from build123d import *

# Parameters (mm, degrees)
F0_R     = 12.5
F0_W     = 5
F0_H     = 20
F1_DEPTH = 25
F2_R     = 15
F3_R     = 5
F4_R     = 2.5
F5_DEPTH = 5
F6_SIZE  = 0.5


with BuildPart() as f1:
    # F0 (on Top) → F1 (new body)
    with BuildSketch(Plane.XY):
        with BuildLine():
            ThreePointArc((-15, 0), (0, -15), (15, 0))
            ThreePointArc((15, 0), (5.352331, 14.012585), (-11.18034, 10))
            ThreePointArc((-11.18034, 10), (-14.012585, 5.352331), (-15, 0))
        make_face()
        Circle(F0_R, mode=Mode.SUBTRACT)
        with BuildLine():
            ThreePointArc((-15, 0), (-14.012585, 5.352331), (-11.18034, 10))
            Line((-11.18034, 10), (-20, 10))
            Line((-20, 10), (-20, 0))
            Line((-20, 0), (-15, 0))
        make_face()
        with Locations((-17.5, -10)):
            Rectangle(F0_W, F0_H)
    extrude(amount=F1_DEPTH)

    # F2
    f2_edges = [f1.edges().sort_by_distance(p)[0] for p in [
        (-11.18034, 10, 12.5),
    ]]
    fillet(f2_edges, radius=F2_R)

    # F3
    f3_edges = [f1.edges().sort_by_distance(p)[0] for p in [
        (-20, 10, 12.5),
    ]]
    fillet(f3_edges, radius=F3_R)

    # F4 (on face) → F5 (cut)
    with BuildSketch(Plane(origin=(-20, 0, 0), x_dir=(0, -1, 0), z_dir=(-1, 0, 0))):
        with Locations((15, 12.5)):
            Circle(F4_R)
    extrude(amount=-F5_DEPTH, mode=Mode.SUBTRACT)

    # F6
    f6_edges = [f1.edges().sort_by_distance(p)[0] for p in [
        (-12.5, 0, 0),
        (-12.5, 0, 25),
    ]]
    chamfer(f6_edges, length=F6_SIZE)


solid = f1.part
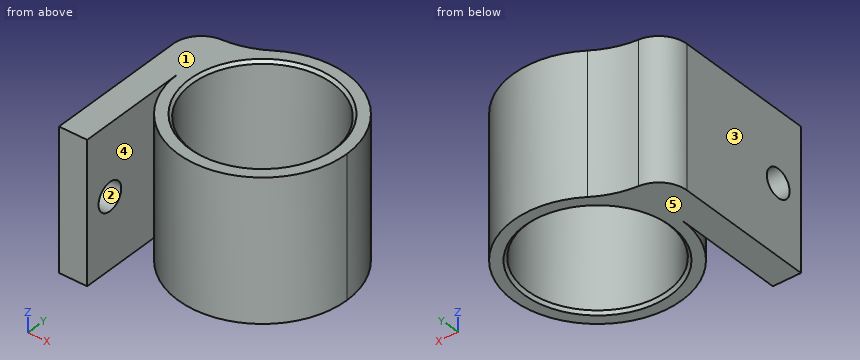
Design review of the part built by this model. Coordinates are the model's own, in mm. Face numbers are marked on the shaded views. A direction names the side the tool comes from. Give positions to 0.01 mm unless a question says otherwise; leave off trailing zeros. Loops run counter-clockwise (first coordinate to the right, second up) from the corner with the lowest first, then second, coordinate; pieces in that order, holes last. Notation, with made-up numbers: (19, -38.75) -> (67, -38.75) arc R6 ccw to (67, -33.75) -> close; hole circle Ø5 at (86.25, 28.5). An arc over 180 degrees is marked (long way). One line per question, with ' | ' between items. Start each with the question number.
(1) Insertion check: P1, Ø4, axis at x = -6, z = 5, coming from the -Y side; P2, Ø1.5, axis at x = -0.5, y = -12, coming from the -Z side; P3, Ø4, axis at y = -15, z = 12.5, coming from the +X side. Each pin has a flat end and moves straight along its axis. Give the tip position at first contact, or say it passes through.
(2) For the marked faces 1 and 2, list the 3-axis set-ups (+Z, -Z, +X, -X, +Y, -Y) from which the entire face can be reached by the end or side of a thin tool; tool diameter is ignored.
(3) For line 1 (Z direction, x = -18.45, y = -15); line 2 (Y direction, x = 0, z = 9); line 3 (X direction, y = 5.5, z = 18.5), list the stretches that pass through material, from the lowest coordinate up.
(4) Draft analysis for pull direction X (two halves, no side actions). For the marked faces 3, 4 and 5, state which applies: +X half, -X half, draft (parallel to the pull), parting line (faces both ways), or undercut.
(5) We need section A-A (x = 0). State the section outline as (y, z) points, and give its area (4 significant figures).
(6) We need section B-B (z = 12.5). State how many separate pieces and enclosed holes the cut face has, and give its area (3 significant figures).
The answers:
1) P1: stops at y = -14.46 | P2: stops at z = 0.24 | P3: stops at x = 7.48
2) face 1: +Z, +X, -X, +Y, -Y | face 2: -X
3) line 1: z = 0 to 10, 15 to 25 | line 2: y = -15 to -12.5, 12.5 to 15 | line 3: x = -19.98 to -11.22, 11.22 to 13.96
4) face 3: -X half | face 4: undercut | face 5: draft
5) outline: (-15, 0) -> (-13, 0) -> (-12.5, 0.5) -> (-12.5, 24.5) -> (-13, 25) -> (-15, 25) -> close; (12.5, 0.5) -> (13, 0) -> (15, 0) -> (15, 25) -> (13, 25) -> (12.5, 24.5) -> close | area: 124.5 mm^2
6) separate pieces: 2 | enclosed holes: 1 | area: 351 mm^2
